Geometry check sheet. Reference: drawing and pictorial views, mm from the part's lowest x, y, z. Coordinates: 2 decimals unless noted, no trailing zeros. Loops run counter-clockwise (first coordinate to the right, second up) from the corner with the lowest first, then second, coordinate; pieces in that order, holes last. Notation, with made-up numbers: M 80,63 L 132,63 A19 ccw 132,100 Z; hole C -6,13 d10. An arc over 180 degrees is marked long. Write each question's results on one line, items separated by ' | '. Start each with the question number.
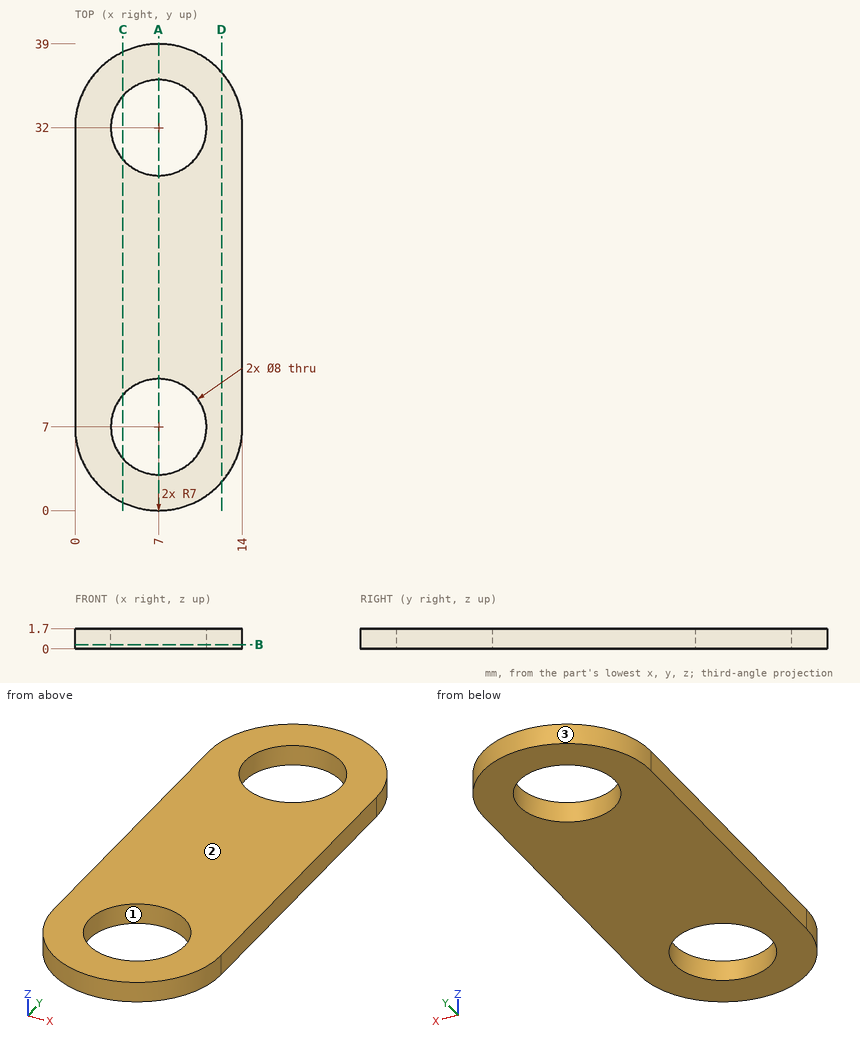
1) Release check for a two-part mould opening along X. For the marked faces 1, 2 and 3 record: +X half, -X half, draft (parallel to the pull), parting line (faces both ways), or undercut.
2) Thickness scan on probe 1 along Y at (x, z) = (7, 0.85); probe 2 along Y at (x, z) = (6, 1.45); probe 3 along X at (y, z) = (32, 0.9). Record the ranges inside material, lowest first.
3) Section check B-B (z = 0.35). Enter the section's corners in (x, y).
4) Section check C-C (x = 4). Enter the section's corners in (y, z).
5) Section check A-A (x = 7). Enter the section's corners in (y, z).
6) Gauge pin test, flat ends, axial feed: P1, Ø1, axis at x = 1.5, z = 0.5, coming from the +Y side; P2, Ø1, axis at x = 8, z = 0.5, coming from the +Y side. Record the tip position at first contact, or that the pin passes through.
7) Section check D-D (x = 12.25). Enter the section's corners in (y, z), then the cut area to 3 significant figures.
Return value:
1) face 1: undercut | face 2: draft | face 3: parting line
2) probe 1: y = 0 to 3, 11 to 28, 36 to 39 | probe 2: y = 0.07 to 3.13, 10.87 to 28.13, 35.87 to 38.93 | probe 3: x = 0 to 3, 11 to 14
3) outline: M 0,7 A7 ccw 14,7 L 14,32 A7 ccw 0,32 Z; hole C 7,7 d8; hole C 7,32 d8
4) outline: M 0.68,0 L 4.35,0 L 4.35,1.7 L 0.68,1.7 Z; M 9.65,0 L 29.35,0 L 29.35,1.7 L 9.65,1.7 Z; M 34.65,0 L 38.32,0 L 38.32,1.7 L 34.65,1.7 Z
5) outline: M 0,0 L 3,0 L 3,1.7 L 0,1.7 Z; M 11,0 L 28,0 L 28,1.7 L 11,1.7 Z; M 36,0 L 39,0 L 39,1.7 L 36,1.7 Z
6) P1: stops at y = 36.9 | P2: stops at y = 38.98
7) outline: M 2.37,0 L 36.63,0 L 36.63,1.7 L 2.37,1.7 Z | area: 58.2 mm2
